from build123d import *


with BuildPart() as part:
    # Sketch1 → Revolve2 (revolve)
    with BuildSketch(Plane.XY, mode=Mode.PRIVATE) as revolve2_sk:
        with BuildLine():
            Line((-55.88, 118.459427374), (-55.88, -33.940572626))
            add(Edge.make_bspline(
                [(-55.88, -33.940572626), (-54.990575769, -80.080925815), (-14.574030728, -85.897657427), (-13.851510687, -95.680738649)],
                knots=[0, 0, 0, 0, 0.984737572, 0.984737572, 0.984737572, 0.984737572], degree=3))
            Line((-13.851510687, -95.680738649), (-13.851510687, -103.52108655))
            Line((-13.851510687, -103.52108655), (-12.889681114, -103.52108655))
            Line((-12.889681114, -103.52108655), (-12.889681114, -95.680738649))
            add(Edge.make_bspline(
                [(-54.922864743, -33.482666024), (-54.019655344, -80.338147614), (-12.354569903, -85.610371161), (-12.889681114, -95.680738649)],
                knots=[0, 0, 0, 0, 1, 1, 1, 1], degree=3))
            Line((-54.922864743, -33.482666024), (-54.922864743, 118.459427374))
            Line((-54.922864743, 118.459427374), (-55.88, 118.459427374))
        make_face()
    revolve(revolve2_sk.sketch.rotate(Axis((0, 76.879343575, 0), (0, -1, 0)), 270), axis=Axis((0, 76.879343575, 0), (0, -1, 0)))


solid = part.part
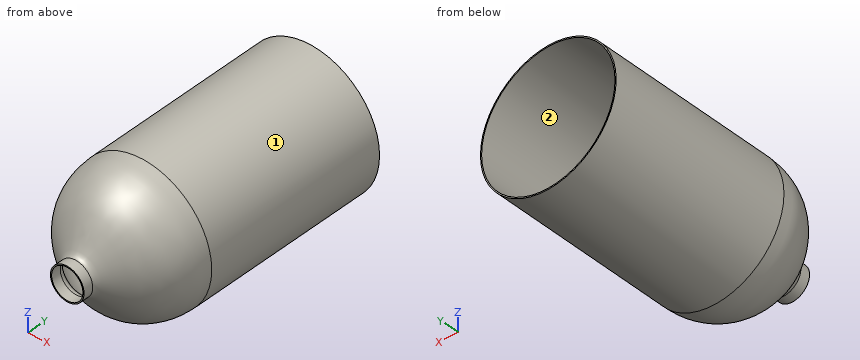
The listing builds one solid part. Answer for the finished solid, in the listing's coordinates (mm). Face numbers are marked on the shaded views. Give positions to 0.01 mm unless a question says otherwise; leave off trailing zeros. Order: outer loops, then holes, each group sorted by start corner. A loop starts at its lowest first (then second) coordinate and runs counter-clockwise, first axis right, second up. Notation, with made-up numbers: (-24.75, 76) - (22.25, 76) arc R18 cw to (22.25, 94) - close; hole circle Ø4 at (-30.75, -5). An arc over 180 degrees is marked (long way). Answer as CSV lines item,"result".
Q1. Determine the mould class of the marked faces 1 and 2 for opening direction Z: pulls with the +Z half, pulls with the -Z half, needs draft (parallel to the pull), parting line crosses it, or undercut.
Answer key:
face 1,"parting line crosses it"
face 2,"undercut"
Q2. Each of these flat-tipped pins is pushed along its axis until it touches: pin 1 Ø1 at (x, z) = (27.5, -31) entering from -Y; pin 2 Ø2 at (x, y) = (38.5, -33.5) entering from +Z; pin 3 Ø1.5 at (x, z) = (-18, 42) entering from -Y. Where does it stop, or does it pass through?
Answer key:
pin 1,"stops at y = -72.76"
pin 2,"stops at z = 41.43"
pin 3,"stops at y = -68.02"
Q3. A cutting plane is placed at A-A, the plane y = -17.5. Determine the outline of the cut face in (x, z).
Answer key:
outline,"circle Ø111.76 at (0, 0); hole circle Ø109.85 at (0, 0)"
Q4. Straight lines are drawn through the part: L1, parallel to X at y = -99.5, z = 0; L2, parallel to X at y = -85, z = -10; L3, parallel to Z at x = 25, y = -39. For each, find the intervals that lie inside material, in ascending order.
Answer key:
L1,"x = -13.85 to -12.89, 12.89 to 13.85"
L2,"x = -23.73 to -21.93, 21.93 to 23.73"
L3,"z = -49.68 to -48.56, 48.56 to 49.68"
